Could you check a few things on this model? Use its own coordinates, in mm. A direction names the side the tool comes from. Give positions to 0.01 mm unless a question says otherwise; leave off trailing zeros. Order: outer loops, then holes, each group sorted by start corner. A loop starts at its lowest first (then second) coordinate and runs counter-clockwise, first axis right, second up. Notation, with made-up numbers: (24.5, 17.5) -> (41.5, 17.5) arc R30 cw to (41.5, 41.5) -> close; hole circle Ø6 at (15, 19). An arc over 180 degrees is marked (long way). Answer as CSV lines item,"result". Start each with the question number.
(1) On a 3-axis mill with a long thin cutter (end or side, diameter ignored), from which of +Z, -Z, +X, -X, +Y, -Y can I reach the whole of each face in a straight line? I mean faces 1 (the face through (19.319, 15.927, 2.535)), 2 (the face through (17.187, -26, 3)), 3 (the face through (14.687, -23, 2)), 4 (the face through (-23, 13.734, 3)). Say none if no direction works.
(2) I need wall thicknesses on L1, parallel to X at y = -2.5, z = 0.95; L2, parallel to X at y = 6, z = 3.1; L3, parallel to Y at x = 3.5, z = 4. Which ranges of each line are inside material? Lowest first, please.
(3) I want a section at B-B (x = -6.5). Please give me the cut outline in (y, z), plus the area to 3 significant figures.
(4) I want a section at C-C (z = 3.2). Give the number of separate pieces and of enclosed holes in the cut face, plus the area to 3 significant figures.
(5) I want a section at A-A (y = -12). Please give me the cut outline in (x, z).
(6) Will these pins go through, and if not, where does the flat tip stop? pin 1 Ø2.5 at (y, z) = (-23.5, 3.5) entering from +X; pin 2 Ø5 at (x, y) = (13.5, -15) entering from +Z; pin 3 Ø3 at (y, z) = (-26, 3) entering from -X; pin 4 Ø1.8 at (y, z) = (20, 3.5) entering from -X.
Autodesk Inventor part; units mm, degrees
ref_plane "YZ Plane" through (0, 0, 0) normal (1, 0, 0) x (0, 1, 0)
ref_plane "XZ Plane" through (0, 0, 0) normal (0, 1, 0) x (-1, 0, 0)
ref_plane "XY Plane" through (0, 0, 0) normal (0, 0, 1) x (1, 0, 0)
sketch "Sketch1" plane through (0, 0, 0) normal (0, 0, 1) x (1, 0, 0)
  line L0 (21.5871, 13.6345) -> (17.0871, 18.1345)
  line L1 (17.0871, 18.1345) -> (-16.7129, 18.1345)
  line L2 (-16.7129, 18.1345) -> (-21.2129, 13.6345)
  line L3 (-21.0966, 13.6345) -> (-21.0966, -20.1655)
  line L4 (21.4709, -20.1655) -> (21.4709, 13.6345)
  line L5 (21.4709, -20.1655) -> (17.0871, -24.4078)
  line L6 (-16.7129, -24.4078) -> (17.0871, -24.4078)
  line L7 (-16.7129, -24.4078) -> (-21.0966, -20.1655)
  line L8 (-24.7129, -28.1655) -> (-24.7129, 13.6345) construction
  line L9 (25.0871, -28.1655) -> (-24.7129, -28.1655) construction
  line L10 (25.0871, -28.1655) -> (25.0871, 13.6345) construction
  line L11 (17.0871, 21.6345) -> (-16.7129, 21.6345) construction
  line L12 (-21.0552, -20.0655) -> (-16.6129, -24.5078)
  line L13 (-16.6129, -24.5078) -> (-16.6129, -28.1655)
  line L14 (-16.6129, -28.1655) -> (17.0871, -28.1655)
  line L15 (25.0871, -20.0655) -> (21.4295, -20.0655)
  line L16 (25.0871, 13.5345) -> (25.0871, -20.0655)
  line L17 (21.4295, 13.5345) -> (25.0871, 13.5345)
  line L18 (21.4295, 13.5345) -> (16.9871, 17.9768)
  line L19 (16.9871, 17.9768) -> (16.9871, 21.6345)
  line L20 (16.9871, 21.6345) -> (-16.6129, 21.6345)
  line L21 (-16.6129, 21.6345) -> (-16.6129, 17.9768)
  line L22 (-16.6129, 17.9768) -> (-21.0552, 13.5345)
  line L23 (-24.7129, 13.5345) -> (-21.0552, 13.5345)
  line L24 (-24.7129, -20.0655) -> (-24.7129, 13.5345)
  line L25 (-21.0552, -20.0655) -> (-24.7129, -20.0655)
  line L26 (-12.3129, -23.2655) -> (12.6871, -23.2655)
  line L27 (12.6871, -23.2655) -> (12.6871, 16.7345)
  line L28 (-12.3129, 16.7345) -> (12.6871, 16.7345)
  line L29 (-12.3129, -23.2655) -> (-12.3129, 16.7345)
  line L30 (14.6871, -25.2655) -> (-14.3129, -25.2655) construction
  line L31 (-14.3129, -25.2655) -> (-14.3129, 18.7345) construction
  line L32 (-14.3129, 18.7345) -> (14.6871, 18.7345) construction
  line L33 (14.6871, 18.7345) -> (14.6871, -25.2655) construction
  line L34 (-17.3129, 21.7345) -> (17.6871, 21.7345) construction
  line L35 (17.6871, 21.7345) -> (17.6871, -28.2655) construction
  line L36 (17.6871, -28.2655) -> (-17.3129, -28.2655) construction
  line L37 (-17.3129, -28.2655) -> (-17.3129, 21.7345) construction
  line L38 (-14.3129, -23.2655) -> (-14.3129, -25.2655)
  line L39 (-14.3129, -25.2655) -> (14.6871, -25.2655)
  line L40 (14.6871, -25.2655) -> (14.6871, -20.0655)
  line L41 (14.6871, -20.0655) -> (17.6871, -20.0655)
  line L42 (17.6871, -20.0655) -> (17.6871, 13.5345)
  line L43 (17.6871, 13.5345) -> (14.6871, 13.5345)
  line L44 (14.6871, 13.5345) -> (14.6871, 18.7345)
  line L45 (14.6871, 18.7345) -> (-14.3129, 18.7345)
  line L46 (-14.3129, 18.7345) -> (-14.3129, 13.5345)
  line L47 (-14.3129, 13.5345) -> (-17.3129, 13.5345)
  line L48 (-17.3129, 13.5345) -> (-17.3129, -20.0655)
  line L49 (-17.3129, -20.0655) -> (-14.3129, -20.0655)
  line L50 (-14.3129, -20.0655) -> (-14.3129, -23.2655)
  line L51 (-16.6129, -28.1655) -> (17.0871, -28.1655)
  line L52 (16.9871, -28.1655) -> (16.9871, -24.3509)
  line L53 (16.9871, -24.3509) -> (21.2726, -20.0655)
  line L54 (21.2726, -20.0655) -> (21.4295, -20.0655)
  point P0 (14.2, -44.8454)
  point P1 (16.9871, 19.8057)
  dimension "d74" = 2
  dimension "d75" = 5
  dimension "d76" = 135
extrude "Extrusion1" add sketch "Sketch1" along normal blind 5 contours L19 L18 L17 L4 L15 L54 L53 L52 L6 L40 L41 L42 L43 L44 L1 | L1 L44 L45 L46 L21 L20 L19 | L46 L47 L48 L49 L50 L38 L6 L12 L25 L3 L23 L22 L21 L1 | L17 L16 L15 L4 | L3 L25 L24 L23 | L6 L52 L14 L13 L12 L38 L39 L40
sketch "Sketch5" plane through (0, 0, 0) normal (0, 0, -1) x (-1, 0, 0)
  line L0 (12.3129, -23.2655) -> (-12.6871, -23.2655) construction
  line L1 (-12.6871, -23.2655) -> (-12.6871, 16.7345) construction
  line L2 (12.3129, 16.7345) -> (-12.6871, 16.7345) construction
  line L3 (12.3129, -23.2655) -> (12.3129, 16.7345) construction
  line L4 (-14.6871, -25.2655) -> (14.3129, -25.2655) construction
  arc A0 (14.3129, -25.2655) -> (-0.1871, -22.4693) centre (0.3594, -58.629) ccw
  arc A1 (12.3827, -25.2655) -> (-0.1871, -23.1694) centre (0.3594, -58.629) ccw
  line L5 (-0.1871, -22.4693) -> (-0.1871, -23.1694)
  line L6 (14.3129, -20.0655) -> (14.3129, -25.2655)
  line L7 (14.3129, -25.2655) -> (12.3827, -25.2655)
  point P0 (0, 0)
  dimension "d79" = 0.7
extrude "Extrusion4" add sketch "Sketch5" against normal up to surface (5 mm away)
mirror "Mirror1" about plane through (0.1871, -23.1694, 0) normal (1, 0, 0) of "Extrusion4"
ref_plane "Work Plane1" through (0.1871, -20.0655, 0) normal (-1, 0, 0) x (0, 0, 1)
ref_plane "Work Plane2" through (-16.6129, -3.2655, 0) normal (0, -1, 0) x (1, 0, 0)
mirror "Mirror2" about plane through (-16.6129, -3.2655, 0) normal (0, -1, 0) of "Extrusion4", "Mirror1"
sketch "Sketch6" plane through (0, 0, 0) normal (0, 0, -1) x (-1, 0, 0)
  spline S0 degree 3 poles (1.425, -3.2655) (1.425, -3.4679) (1.3845, -3.6839) (1.22, -4.081) (1.0959, -4.2623) (0.8097, -4.5486) (0.6284, -4.6726) (0.2312, -4.8371) (0.0153, -4.8776) (-0.3896, -4.8776) (-0.6055, -4.8371) (-1.0027, -4.6726) (-1.1839, -4.5486) (-1.4702, -4.2623) (-1.5943, -4.081) (-1.7588, -3.6839) (-1.7992, -3.4679) (-1.7992, -3.0631) (-1.7588, -2.8471) (-1.5943, -2.45) (-1.4702, -2.2687) (-1.1839, -1.9824) (-1.0027, -1.8584) (-0.6055, -1.6939) (-0.3896, -1.6534) (0.0153, -1.6534) (0.2312, -1.6939) (0.6284, -1.8584) (0.8097, -1.9824) (1.0959, -2.2687) (1.22, -2.45) (1.3845, -2.8471) (1.425, -3.0631) (1.425, -3.2655) knots 0 0 0 0 0.060733 0.060733 0.121465 0.121465 0.182198 0.182198 0.24293 0.24293 0.303663 0.303663 0.364395 0.364395 0.425128 0.425128 0.48586 0.48586 0.546593 0.546593 0.607326 0.607326 0.668058 0.668058 0.728791 0.728791 0.789523 0.789523 0.850256 0.850256 0.910988 0.910988 0.971721 0.971721 0.971721 0.971721
  line L0 (17.3129, 13.5345) -> (17.3129, -20.0655)
  arc A0 (13.2973, -3.2655) -> (17.3129, -20.0655) centre (48.9305, -3.6282) ccw
  line L1 (17.3129, -20.0655) -> (14.3129, -20.0655)
  arc A1 (11.9598, -3.2655) -> (15.8129, -20.0655) centre (48.9305, -3.6282) ccw
  line L2 (11.9598, -3.2655) -> (13.2973, -3.2655)
  line L3 (15.8129, -20.0655) -> (17.3129, -20.0655)
  point P0 (0, 0)
  point P1 (1.425, -3.2655)
extrude "Extrusion5" add sketch "Sketch6" against normal up to surface (5 mm away) contours A0 L1 A1 L2
mirror "Mirror3" about plane through (-11.9598, -3.2655, 0) normal (0, 1, 0) of "Extrusion5"
mirror "Mirror4" about plane through (0.1871, -20.0655, 0) normal (-1, 0, 0) of "Extrusion5", "Mirror3"
sketch "Skizze7" plane through (0, 0, 5) normal (0, 0, 1) x (1, 0, 0)
  arc A0 (12.3341, -3.2655) -> (16.1871, -20.0655) centre (49.3047, -3.6282) ccw construction
  line L0 (16.1871, -20.0655) -> (14.6871, -20.0655)
  line L1 (14.6871, -20.0655) -> (14.6871, -25.2655)
  arc A1 (14.6871, -25.2655) -> (0.1871, -22.4693) centre (0.7336, -58.629) ccw construction
  arc A2 (0.1871, -22.4693) -> (-14.3129, -25.2655) centre (-0.3594, -58.629) ccw construction
  line L2 (-14.3129, -25.2655) -> (-14.3129, -20.0655) construction
  line L3 (-14.3129, -20.0655) -> (-15.8129, -20.0655) construction
  arc A3 (-15.8129, -20.0655) -> (-11.9598, -3.2655) centre (-48.9305, -3.6282) ccw construction
  arc A4 (-11.9598, -3.2655) -> (-15.8129, 13.5345) centre (-48.9305, -2.9028) ccw construction
  line L4 (-15.8129, 13.5345) -> (-14.3129, 13.5345) construction
  line L5 (-14.3129, 13.5345) -> (-14.3129, 18.7345) construction
  arc A5 (-14.3129, 18.7345) -> (0.1871, 15.9383) centre (-0.3594, 52.098) ccw construction
  arc A6 (0.1871, 15.9383) -> (14.6871, 18.7345) centre (0.7336, 52.098) ccw construction
  line L6 (14.6871, 18.7345) -> (14.6871, 13.5345) construction
  line L7 (14.6871, 13.5345) -> (16.1871, 13.5345) construction
  arc A7 (16.1871, 13.5345) -> (12.3341, -3.2655) centre (49.3047, -2.9028) ccw construction
  arc A8 (-17.3129, -20.0655) -> (-13.2973, -3.2655) centre (-48.9305, -3.6282) ccw construction
  line L8 (-17.3129, -20.0655) -> (-17.3129, 13.5345) construction
  arc A9 (-13.2973, -3.2655) -> (-17.3129, 13.5345) centre (-48.9305, -2.9028) ccw construction
  arc A10 (17.6871, 13.5345) -> (13.6715, -3.2655) centre (49.3047, -2.9028) ccw construction
  line L9 (17.6871, 13.5345) -> (17.6871, -20.0655) construction
  arc A11 (13.6715, -3.2655) -> (17.6871, -20.0655) centre (49.3047, -3.6282) ccw construction
  line L10 (12.757, -25.2655) -> (-12.3827, -25.2655) construction
  arc A12 (0.1871, -23.1694) -> (-12.3827, -25.2655) centre (-0.3594, -58.629) ccw construction
  arc A13 (12.757, -25.2655) -> (0.1871, -23.1694) centre (0.7336, -58.629) ccw construction
  arc A14 (0.1871, 16.6384) -> (12.757, 18.7345) centre (0.7336, 52.098) ccw construction
  arc A15 (-12.3827, 18.7345) -> (0.1871, 16.6384) centre (-0.3594, 52.098) ccw construction
  line L11 (-12.3827, 18.7345) -> (12.757, 18.7345) construction
  line L12 (-21.0552, -20.0655) -> (-16.6129, -24.5078)
  line L13 (-16.6129, -24.5078) -> (-16.6129, -28.1655)
  line L14 (-16.6129, -28.1655) -> (16.9871, -28.1655) construction
  line L15 (16.9871, -28.1655) -> (16.9871, -24.3509)
  line L16 (16.9871, -24.3509) -> (21.2726, -20.0655)
  line L17 (21.2726, -20.0655) -> (25.0871, -20.0655)
  line L18 (25.0871, -20.0655) -> (25.0871, 13.5345) construction
  line L19 (25.0871, 13.5345) -> (21.4295, 13.5345)
  line L20 (21.4295, 13.5345) -> (16.9871, 17.9768)
  line L21 (16.9871, 17.9768) -> (16.9871, 21.6345)
  line L22 (16.9871, 21.6345) -> (-16.6129, 21.6345) construction
  line L23 (-16.6129, 21.6345) -> (-16.6129, 17.9768)
  line L24 (-16.6129, 17.9768) -> (-21.0552, 13.5345)
  line L25 (-21.0552, 13.5345) -> (-24.7129, 13.5345)
  line L26 (-24.7129, 13.5345) -> (-24.7129, -20.0655) construction
  line L27 (-24.7129, -20.0655) -> (-21.0552, -20.0655)
  line L28 (-16.8129, 21.8345) -> (17.1871, 21.8345) construction
  line L29 (17.1871, 21.8345) -> (17.1871, 18.0597)
  line L30 (17.1871, 18.0597) -> (21.5123, 13.7345)
  line L31 (21.5123, 13.7345) -> (25.2871, 13.7345)
  line L32 (25.2871, 13.7345) -> (25.2871, -20.2655) construction
  line L33 (25.2871, -20.2655) -> (21.3554, -20.2655)
  line L34 (21.3554, -20.2655) -> (17.1871, -24.4338)
  line L35 (17.1871, -24.4338) -> (17.1871, -28.3655)
  line L36 (17.1871, -28.3655) -> (-16.8129, -28.3655) construction
  line L37 (-16.8129, -28.3655) -> (-16.8129, -24.5907)
  line L38 (-16.8129, -24.5907) -> (-21.1381, -20.2655)
  line L39 (-21.1381, -20.2655) -> (-24.9129, -20.2655)
  line L40 (-24.9129, -20.2655) -> (-24.9129, 13.7345) construction
  line L41 (-24.9129, 13.7345) -> (-21.1381, 13.7345)
  line L42 (-21.1381, 13.7345) -> (-16.8129, 18.0597)
  line L43 (-16.8129, 18.0597) -> (-16.8129, 21.8345)
  line L44 (-21.0552, 13.5345) -> (-24.7129, 13.5345)
  line L45 (-24.7129, 13.5345) -> (-24.7129, 13.7345)
  line L46 (-16.6129, 21.6345) -> (-16.8129, 21.6345)
  line L47 (16.9871, 17.9768) -> (16.9871, 21.6345)
  line L48 (16.9871, 21.6345) -> (17.1871, 21.6345)
  line L49 (25.0871, -20.0655) -> (25.0871, 13.5345)
  line L50 (25.0871, 13.5345) -> (25.0871, 13.7345)
  line L51 (25.0871, -20.0655) -> (25.0871, -20.2655)
  line L52 (-16.6129, -28.1655) -> (16.9871, -28.1655)
  line L53 (16.9871, -28.1655) -> (17.1871, -28.1655)
  line L54 (-16.6129, -28.1655) -> (-16.8129, -28.1655)
  line L55 (-24.7129, -20.0655) -> (-24.7129, -20.2655)
  point P0 (0, 0)
  dimension "d83" = 0.2
extrude "IM_offset" add sketch "Skizze7" against normal up to surface (5 mm away)
properties part number "20_Cube_Insert_Lens_Cylindrical_v3"
Final values:
1,face 1,"+Z, -Z, +X, +Y"
1,face 2,"+Z, -Z, +X, -Y"
1,face 3,"+Z, -Z"
1,face 4,"+Z, -Z, -X, +Y"
2,L1,"-24.71 to -17.31, -13.3 to -11.96, 12.33 to 13.67, 17.69 to 25.09"
2,L2,"-24.71 to -17.31, -14.43 to -13.05, 13.42 to 14.8, 17.69 to 25.09"
2,L3,"-28.17 to -25.27, -23.27 to -22.57, 16.04 to 16.74, 18.73 to 21.63"
3,outline,"(-28.17, 0) -> (-25.27, 0) -> (-25.27, 5) -> (-28.17, 5) -> close; (-23.7, 0) -> (-22.99, 0) -> (-22.99, 5) -> (-23.7, 5) -> close; (16.46, 0) -> (17.17, 0) -> (17.17, 5) -> (16.46, 5) -> close; (18.73, 0) -> (21.63, 0) -> (21.63, 5) -> (18.73, 5) -> close"
3,area,"36.1 mm²"
4,separate pieces,"1"
4,enclosed holes,"5"
4,area,"922 mm²"
5,outline,"(-24.71, 0) -> (-17.31, 0) -> (-17.31, 5) -> (-24.71, 5) -> close; (-14.29, 0) -> (-12.92, 0) -> (-12.92, 5) -> (-14.29, 5) -> close; (13.29, 0) -> (14.67, 0) -> (14.67, 5) -> (13.29, 5) -> close; (17.69, 0) -> (25.09, 0) -> (25.09, 5) -> (17.69, 5) -> close"
6,pin 1,"x = 19.37"
6,pin 2,"z = 5"
6,pin 3,"x = -16.9"
6,pin 4,"x = -16.81"
